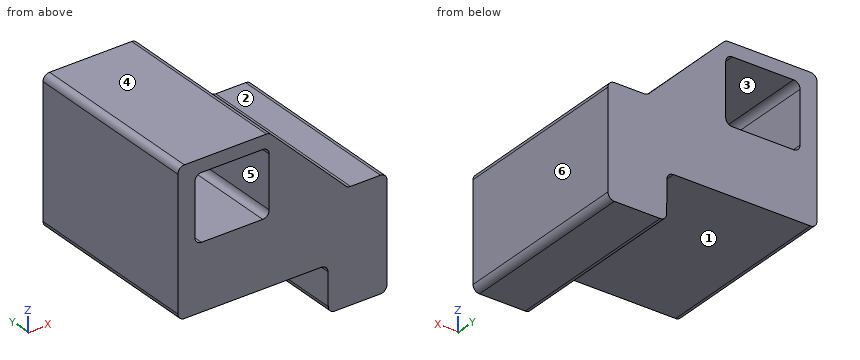
from build123d import *

# Parameters (mm, degrees)
F1_DEPTH = 70
F3_DEPTH = 140.001
F4_R     = 5


with BuildPart() as f1:
    # F0 (on Front) → F1 (new body, symmetric)
    with BuildSketch(Plane.XZ):
        Polygon((-70, 142.023449), (-70, 32.023449), (45, 32.023449), (45.334238, -2.976551), (90.334238, -2.976551), (90.334238, 82.023449), (60.334238, 82.023449), (0, 142.023449), align=None)
    extrude(amount=F1_DEPTH, both=True)

    # F2 (on face) → F3 (cut, through all)
    with BuildSketch(Plane(origin=(0, 70, 0), x_dir=(-1, 0, 0), z_dir=(0, 1, 0))):
        with BuildLine():
            Line((52, 132.023449), (5, 132.023449))
            ThreePointArc((5, 132.023449), (1.464466, 130.558983), (0, 127.023449))
            Line((0, 127.023449), (0, 87.023449))
            ThreePointArc((0, 87.023449), (1.464466, 83.487915), (5, 82.023449))
            Line((5, 82.023449), (52, 82.023449))
            ThreePointArc((52, 82.023449), (55.535534, 83.487915), (57, 87.023449))
            Line((57, 87.023449), (57, 127.023449))
            ThreePointArc((57, 127.023449), (55.535534, 130.558983), (52, 132.023449))
        make_face()
    extrude(amount=-F3_DEPTH, mode=Mode.SUBTRACT)

    # F4
    f4_edges = [f1.edges().sort_by_distance(p)[0] for p in [
        (0, 0, 142.023449),
        (60.334238, 0, 82.023449),
        (90.334238, 0, 82.023449),
        (90.334238, 0, -2.976551),
        (45.334238, 0, -2.976551),
        (45, 0, 32.023449),
        (-70, 0, 32.023449),
        (-70, 0, 142.023449),
    ]]
    fillet(f4_edges, radius=F4_R)


solid = f1.part
Model file for the job. Use its own axes, mm. Face numbers are marked on the shaded views. A direction names the side the tool comes from. Give positions to 0.01 mm unless a question says otherwise; leave off trailing zeros. Order: outer loops, then holes, each group sorted by start corner. A loop starts at its lowest first (then second) coordinate and runs counter-clockwise, first axis right, second up. Notation, with made-up numbers: M 59,-25.75 L 113,-25.75 A11 cw 113,-7.75 Z; hole C 13.25,7 d11. An arc over 180 degrees is marked long. Write item = value, one per line.
Q1. Cut at B-B, the plane z = 113.5. List the corners of the cut face in (x, y), then the cut area to 3 significant figures.
Derived:
outline = M -70,-70 L -57,-70 L -57,70 L -70,70 Z; M 0,-70 L 28.68,-70 L 28.68,70 L 0,70 Z
area = 5,840 mm2
Q2. Cut at A-A, the plane x = -7.5. List the corners of the cut face in (y, z).
Derived:
outline = M -70,32.02 L 70,32.02 L 70,82.02 L -70,82.02 Z; M -70,132.02 L 70,132.02 L 70,142.02 L -70,142.02 Z
Q3. Drill centre lines: line 1 (Z direction, x = -51, y = 15); line 2 (X direction, y = 49.5, z = 97); line 3 (Z direction, x = 78.5, y = -9). Where is each one in solid material? Low to high. Write a range as [from, to].
Derived:
line_1 = [32.02, 82.02], [132.02, 142.02]
line_2 = [-70, -57], [0, 45.27]
line_3 = [-2.98, 82.02]
Q4. Cut at C-C, the plane y = -57. List the corners of the cut face in (x, z), then the cut area to 3 significant figures.
Derived:
outline = M -70,37.02 A5 ccw -65,32.02 L 40.05,32.02 A5 cw 45.05,27.07 L 45.29,1.98 A5 ccw 50.29,-2.98 L 85.33,-2.98 A5 ccw 90.33,2.02 L 90.33,77.02 A5 ccw 85.33,82.02 L 62.4,82.02 A5 cw 58.87,83.48 L 1.46,140.57 A5 ccw -2.06,142.02 L -65,142.02 A5 ccw -70,137.02 Z; hole M -57,87.02 A5 ccw -52,82.02 L -5,82.02 A5 ccw 0,87.02 L 0,127.02 A5 ccw -5,132.02 L -52,132.02 A5 ccw -57,127.02 Z
area = 12,800 mm2
Q5. Flat gauge pins, fed straight in: pin 1 (12 mm diameter, centred on y = -6.5, z = 106, fed in from +X); pin 2 (6 mm diameter, centred on y = -16, z = 16, fed in from -X); pin 3 (1.5 mm diameter, centred on x = 18.5, y = -1.5, fed in from -Z). Where does each tip first touch, or does it go through?
Derived:
pin_1 = 42.26
pin_2 = 45.12
pin_3 = 32.02
Q6. Two-plate mould, pull along Z, no slides. Class the marked faces 4, 5 and 6: pulls with the +Z half, pulls with the -Z half, needs draft (parallel to the pull), parting line crosses it, or undercut.
Derived:
face_4 = pulls with the +Z half
face_5 = undercut
face_6 = needs draft
Q7. Cut at D-D, the plane x = 48. List the corners of the cut face in (y, z).
Derived:
outline = M -70,-2.42 L 70,-2.42 L 70,94.29 L -70,94.29 Z
Q8. Tool access for the marked faces 1, 2 and 3: list every direction of +Z, -Z, +X, -X, +Y, -Y with a clear straight run to the whole face (end or side of a thin tool).
Derived:
face_1 = -Z, -X, +Y, -Y
face_2 = +Z, +X, +Y, -Y
face_3 = +Y, -Y
